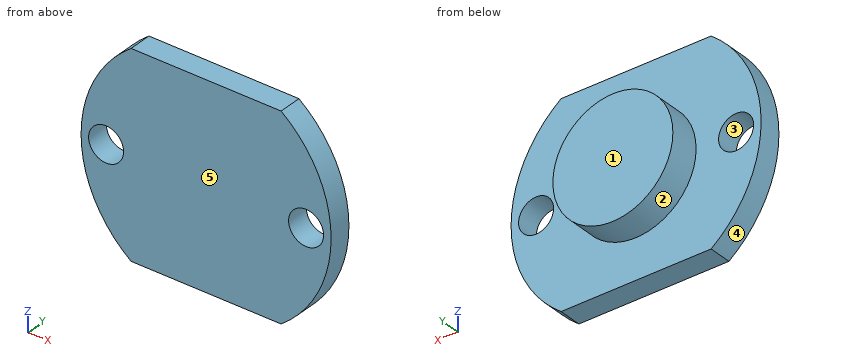
from build123d import *

# Parameters (mm, degrees)
SKETCH1_R           = 1.75
BOSS_EXTRUDE1_DEPTH = 2.3
SKETCH3_R           = 6
BOSS_EXTRUDE2_DEPTH = 3


with BuildPart() as part:
    # Sketch1 → Boss-Extrude1 (new body)
    with BuildSketch(Plane(origin=(0, 0, 0), x_dir=(1, 0, 0), z_dir=(0, 1, 0))):
        with BuildLine():
            Line((7.5, -10), (-7.5, -10))
            ThreePointArc((-7.5, -10), (-12.5, 0), (-7.5, 10))
            Line((-7.5, 10), (7.5, 10))
            ThreePointArc((7.5, 10), (12.5, 0), (7.5, -10))
        make_face()
        with Locations((10, 0)):
            Circle(SKETCH1_R, mode=Mode.SUBTRACT)
        with Locations((-10, 0)):
            Circle(SKETCH1_R, mode=Mode.SUBTRACT)
    extrude(amount=BOSS_EXTRUDE1_DEPTH)

    # Sketch3 → Boss-Extrude2 (add)
    with BuildSketch(Plane(origin=(0, 2.3, 0), x_dir=(1, 0, 0), z_dir=(0, 1, 0))):
        Circle(SKETCH3_R)
    extrude(amount=BOSS_EXTRUDE2_DEPTH)


solid = part.part
The listing builds one solid part. Answer for the finished solid, in the listing's coordinates (mm). Face numbers are marked on the shaded views. A direction names the side the tool comes from. Give positions to 0.01 mm unless a question says otherwise; leave off trailing zeros. Write each loop counter-clockwise with the first axis right and the second up, starting at its lowest first coordinate (ties: lowest second). Pieces come first, ordered by that corner, then holes.
1) Given P1, Ø2, axis at x = 10, z = 0, coming from the -Y side; P2, Ø3, axis at y = 4, z = -4, coming from the -X side, each flat-ended and moving along its own axis, determine where each tip first touches the part or whether it passes through.
2) Section C-C (x = 0) is taken. Write down the section's boundary in (y, z).
3) For a pull along Z with two mould halves and no side action, classify the marked faces 3, 4 and 5 as pulls with the +Z half, pulls with the -Z half, needs draft (parallel to the pull), parting line crosses it, or undercut.
4) Section A-A (x = 10) is taken. Write down the section's boundary in (y, z), and give its area (4 significant figures).
5) A tool of negligible diameter and unlimited length cuts with its end or side. For the marked faces 1 and 2, from which of +Z, -Z, +X, -X, +Y, -Y can it reach the whole face along a straight path? Write none if from no direction.
6) Find the intervals of material crossed by L1, parallel to Z at x = -10, y = 0.6; L2, parallel to Y at x = 11.75, z = 4; L3, parallel to Z at x = 11.25, y = 2.2, in increasing order.
7) Section D-D (y = 1.25) is taken. Write down the section's boundary in (x, z).
8) Section B-B (z = 0) is taken. Write down the section's boundary in (x, y), and give its area (3 significant figures).
Response:
1. P1: passes through
1. P2: stops at x = -5.45
2. outline: (0, -10) - (2.3, -10) - (2.3, -6) - (5.3, -6) - (5.3, 6) - (2.3, 6) - (2.3, 10) - (0, 10) - close
3. face 3: undercut
3. face 4: parting line crosses it
3. face 5: needs draft
4. outline: (0, -7.5) - (2.3, -7.5) - (2.3, -1.75) - (0, -1.75) - close; (0, 1.75) - (2.3, 1.75) - (2.3, 7.5) - (0, 7.5) - close
4. area: 26.45 mm2
5. face 1: +Z, -Z, +X, -X, +Y
5. face 2: +Y
6. L1: z = -7.5 to -1.75, 1.75 to 7.5
6. L2: y = 0 to 2.3
6. L3: z = -5.45 to -1.22, 1.22 to 5.45
7. outline: (-7.5, -10) - (7.5, -10) arc R12.5 ccw to (7.5, 10) - (-7.5, 10) arc R12.5 ccw to start; hole circle Ø3.5 at (-10, 0); hole circle Ø3.5 at (10, 0)
8. outline: (-12.5, 0) - (-11.75, 0) - (-11.75, 2.3) - (-12.5, 2.3) - close; (-8.25, 0) - (8.25, 0) - (8.25, 2.3) - (6, 2.3) - (6, 5.3) - (-6, 5.3) - (-6, 2.3) - (-8.25, 2.3) - close; (11.75, 0) - (12.5, 0) - (12.5, 2.3) - (11.75, 2.3) - close
8. area: 77.4 mm2
